```python
from build123d import *

# Parameters (mm, degrees)
ESQUISSE1_W             = 17.2
ESQUISSE1_H             = 17.2
BOSS_EXTRU_1_DEPTH      = 5
ESQUISSE2_R             = 1
BOSS_EXTRU_2_DEPTH      = 5
ESQUISSE3_R             = 14.2
BOSS_EXTRU_3_DEPTH      = 7.8
ESQUISSE4_R             = 15
BOSS_EXTRU_4_DEPTH      = 7
ESQUISSE5_R             = 14
BOSS_EXTRU_5_DEPTH      = 2.5
ESQUISSE6_R             = 15
BOSS_EXTRU_6_DEPTH      = 11.5
ESQUISSE7_R             = 14.2
BOSS_EXTRU_7_DEPTH      = 2
ESQUISSE8_R             = 15
BOSS_EXTRU_8_DEPTH      = 7
ESQUISSE9_R             = 14
ENL_V_MAT_EXTRU_1_DEPTH = 1.5
ESQUISSE10_R            = 10
ENL_V_MAT_EXTRU_2_DEPTH = 1.5
CHANFREIN1_SIZE         = 1


with BuildPart() as part:
    # Esquisse1 → Boss.-Extru.1 (new body)
    with BuildSketch(Plane(origin=(0, 0, 0), x_dir=(0, 0, -1), z_dir=(1, 0, 0))):
        Rectangle(ESQUISSE1_W, ESQUISSE1_H)
    extrude(amount=BOSS_EXTRU_1_DEPTH)

    # Esquisse2 → Boss.-Extru.2 (add)
    with BuildSketch(Plane(origin=(0, 0, 0), x_dir=(0, 0, -1), z_dir=(1, 0, 0))):
        with BuildLine():
            Line((-2, 8.6), (-2, 10))
            ThreePointArc((-2, 10), (0, 12), (2, 10))
            Line((2, 10), (2, 8.6))
            Line((2, 8.6), (-2, 8.6))
        make_face()
        with Locations((0, 10)):
            Circle(ESQUISSE2_R, mode=Mode.SUBTRACT)
    boss_extru_2 = extrude(amount=BOSS_EXTRU_2_DEPTH)

    # Symétrie1: Boss.-Extru.2 across plane
    add(boss_extru_2.mirror(Plane.ZX))

    # Esquisse3 → Boss.-Extru.3 (add)
    with BuildSketch(Plane(origin=(5, 0, 0), x_dir=(0, 0, -1), z_dir=(1, 0, 0))):
        Circle(ESQUISSE3_R)
    extrude(amount=BOSS_EXTRU_3_DEPTH)

    # Esquisse4 → Boss.-Extru.4 (add)
    with BuildSketch(Plane(origin=(12.8, 0, 0), x_dir=(0, 0, -1), z_dir=(1, 0, 0))):
        Circle(ESQUISSE4_R)
    extrude(amount=BOSS_EXTRU_4_DEPTH)

    # Esquisse5 → Boss.-Extru.5 (add)
    with BuildSketch(Plane(origin=(19.8, 0, 0), x_dir=(0, 0, -1), z_dir=(1, 0, 0))):
        Circle(ESQUISSE5_R)
    extrude(amount=BOSS_EXTRU_5_DEPTH)

    # Esquisse6 → Boss.-Extru.6 (add)
    with BuildSketch(Plane(origin=(22.3, 0, 0), x_dir=(0, 0, -1), z_dir=(1, 0, 0))):
        Circle(ESQUISSE6_R)
    extrude(amount=BOSS_EXTRU_6_DEPTH)

    # Esquisse7 → Boss.-Extru.7 (add)
    with BuildSketch(Plane(origin=(33.8, 0, 0), x_dir=(0, 0, -1), z_dir=(1, 0, 0))):
        Circle(ESQUISSE7_R)
    extrude(amount=BOSS_EXTRU_7_DEPTH)

    # Esquisse8 → Boss.-Extru.8 (add)
    with BuildSketch(Plane(origin=(35.8, 0, 0), x_dir=(0, 0, -1), z_dir=(1, 0, 0))):
        Circle(ESQUISSE8_R)
    extrude(amount=BOSS_EXTRU_8_DEPTH)

    # Esquisse9 → Enlèv. mat.-Extru.1 (cut)
    with BuildSketch(Plane(origin=(42.8, 0, 0), x_dir=(0, 0, -1), z_dir=(1, 0, 0))):
        Circle(ESQUISSE9_R)
    extrude(amount=-ENL_V_MAT_EXTRU_1_DEPTH, mode=Mode.SUBTRACT)

    # Esquisse10 → Enlèv. mat.-Extru.2 (cut)
    with BuildSketch(Plane(origin=(41.3, 0, 0), x_dir=(0, 0, -1), z_dir=(1, 0, 0))):
        Circle(ESQUISSE10_R)
    extrude(amount=-ENL_V_MAT_EXTRU_2_DEPTH, mode=Mode.SUBTRACT)

    # Chanfrein1
    chanfrein1_edges = [part.edges().sort_by_distance(p)[0] for p in [
        (41.3, 0, 10),
    ]]
    chamfer(chanfrein1_edges, length=CHANFREIN1_SIZE)


solid = part.part
```
CAD build for the part. Positions are in the model's coordinates, mm. A direction names the side the tool comes from. Coordinates: 2 decimals unless noted, no trailing zeros. Order: outer loops, then holes, each group sorted by start corner. A loop starts at its lowest first (then second) coordinate and runs counter-clockwise, first axis right, second up. Notation, with made-up numbers: M 0.5,26 L 57.5,26 A24 cw 57.5,59 Z; hole C 71,-2.75 d10. An arc over 180 degrees is marked long. Answer as CSV lines item,"result".
1) Cut at B-B (z = 13.25). List the corners of the cut face in (x, y).
Verdict:
outline,"M 5,-5.11 L 12.8,-5.11 L 12.8,-7.03 L 19.8,-7.03 L 19.8,-4.52 L 22.3,-4.52 L 22.3,-7.03 L 33.8,-7.03 L 33.8,-5.11 L 35.8,-5.11 L 35.8,-7.03 L 42.8,-7.03 L 42.8,-4.52 L 41.3,-4.52 L 41.3,4.52 L 42.8,4.52 L 42.8,7.03 L 35.8,7.03 L 35.8,5.11 L 33.8,5.11 L 33.8,7.03 L 22.3,7.03 L 22.3,4.52 L 19.8,4.52 L 19.8,7.03 L 12.8,7.03 L 12.8,5.11 L 5,5.11 Z"
2) Cut at A-A (x = 34.5). List the corners of the cut face in (y, z).
Verdict:
outline,"C 0,0 d28.4"
3) Mould opens along Y. For faces 1 (the cylindrical face through (21.032, -5.362, -12.932)), 2 (the cylindrical face through (2, -12, 0)), 3 (the flat face through (39.8, 0, 0)), 4 (the flat face through (2, 8.6, 5)) say: released by +Y, released by -Y, zero draft, split by the parting line, or undercut.
Verdict:
face 1,"split by the parting line"
face 2,"released by -Y"
face 3,"undercut"
face 4,"released by +Y"
4) Flat gauge pins, fed straight in: P1, Ø2, axis at x = 22, z = -4.5, coming from the +Y side; P2, Ø1.5, axis at x = 3.5, y = -0.5, coming from the -Z side; P3, Ø8.5, axis at y = 3.5, z = -2, coming from the +X side. Where does each tip first touch, or does it go through?
Verdict:
P1,"y = 14.57"
P2,"z = -8.6"
P3,"x = 39.8"
5) Cut at C-C (x = 26). List the corners of the cut face in (y, z), then the cut area to 3 significant figures.
Verdict:
outline,"C 0,0 d30"
area,"707 mm2"
6) Drill centre lines: L1, parallel to Y at x = 1.95, z = 0; L2, parallel to X at y = -12.5, z = 6.5; L3, parallel to Y at x = 41.9, z = 0. Where is each one in solid material? Low to high. Write a range as from..to.
Verdict:
L1,"-12..-11, -9..9, 11..12"
L2,"5..19.8, 22.3..42.8"
L3,"-15..-14, 14..15"
7) 3-axis set-ups, long thin cutter, end or side, ignore diameter. For faces 5 (the flat face through (41.3, -9.3, -6.2)), 6 (the flat face through (12.8, -13.3, -5.5)), 7 (the flat face through (2, -8.6, 5)), 8 (the flat face through (2, -9, -2)): which of +Z, -Z, +X, -X, +Y, -Y reach the whole face in a straight line?
Verdict:
face 5,"+X"
face 6,"-X"
face 7,"+Z, -X, -Y"
face 8,"-Z, -X, -Y"
8) Cut at D-D (z = -13). List the corners of the cut face in (x, y), then the cut area to 3 significant figures.
Verdict:
outline,"M 5,-5.71 L 12.8,-5.71 L 12.8,-7.48 L 19.8,-7.48 L 19.8,-5.2 L 22.3,-5.2 L 22.3,-7.48 L 33.8,-7.48 L 33.8,-5.71 L 35.8,-5.71 L 35.8,-7.48 L 42.8,-7.48 L 42.8,-5.2 L 41.3,-5.2 L 41.3,5.2 L 42.8,5.2 L 42.8,7.48 L 35.8,7.48 L 35.8,5.71 L 33.8,5.71 L 33.8,7.48 L 22.3,7.48 L 22.3,5.2 L 19.8,5.2 L 19.8,7.48 L 12.8,7.48 L 12.8,5.71 L 5,5.71 Z"
area,"504 mm2"
